```python
from build123d import *

# Parameters (mm, degrees)
SKETCH030_R             = 10
SKETCH030_R_2           = 1.55
SKETCH030_R_3           = 1.25
PAD027_DEPTH            = 2.5
SKETCH031_R             = 4.5
SKETCH031_R_2           = 3
PAD028_DEPTH            = 2
SKETCH032_R             = 3
POCKET009_DEPTH         = 1
BODY011_PLACEMENT_ANGLE = 180


with BuildPart() as part:
    # Sketch030 → Pad027 (new body)
    with BuildSketch(Plane.YZ):
        Circle(SKETCH030_R)
        Circle(SKETCH030_R_2, mode=Mode.SUBTRACT)
        with Locations((-7.35, 0)):
            Circle(SKETCH030_R_3, mode=Mode.SUBTRACT)
        with Locations((0, -7.35)):
            Circle(SKETCH030_R_3, mode=Mode.SUBTRACT)
        with Locations((7.35, 0)):
            Circle(SKETCH030_R_3, mode=Mode.SUBTRACT)
        with Locations((0, 7.35)):
            Circle(SKETCH030_R_3, mode=Mode.SUBTRACT)
    extrude(amount=PAD027_DEPTH)

    # Sketch031 (on Face8 of Pad027) → Pad028 (join)
    with BuildSketch(Plane.YZ.offset(2.5)):
        Circle(SKETCH031_R)
        Circle(SKETCH031_R_2, mode=Mode.SUBTRACT)
    extrude(amount=PAD028_DEPTH)

    # Sketch032 (on Face10 of Pad028) → Pocket009 (cut)
    with BuildSketch(Plane.YZ.offset(2.5)):
        Circle(SKETCH032_R)
    extrude(amount=-POCKET009_DEPTH, mode=Mode.SUBTRACT)


with BuildPart() as part_1:
    # Body011 placement: moved
    add(part.part.moved(Location((19.2, 11.3, 0))).rotate(Axis((19.2, 11.3, 0), (0, 0, 1)), BODY011_PLACEMENT_ANGLE))


solid = part_1.part
```
Design review of the part built by this model. Coordinates are the model's own, in mm. Coordinates: 2 decimals unless noted, no trailing zeros. Write each loop counter-clockwise with the first axis right and the second up, starting at its lowest first coordinate (ties: lowest second). Pieces come first, ordered by that corner, then holes.
1) Insertion check: pin 1 (4 mm diameter, centred on y = 11.3, z = 7.35, fed in from -X); pin 2 (1.8 mm diameter, centred on y = 11.5, z = 0.5, fed in from -X); pin 3 (1 mm diameter, centred on x = 18, z = -7, fed in from +Y). Each pin has a flat end and moves straight along its axis. Give the tip position at first contact, or say it passes through.
2) Add section D-D (z = 7.35). Write out the cut boundary in (x, y).
3) Add section B-B (y = 11.3). Write out the cut boundary in (x, z), plus the area to 4 significant figures.
4) Add section C-C (y = 3.95). Write out the cut boundary in (x, z).
5) Add section A-A (z = 0). Write out the cut boundary in (x, y).
6) To check wall thickness, follow L1, parallel to Z at x = 17.3, y = 11.3; L2, parallel to Y at x = 18.45, z = 1; L3, parallel to X at y = 8, z = 6. State the ranges of each line that lie inside material, in increasing order.
7) Mouldability with a two-part tool opening along Y and no side actions: class faces 1 (the cylindrical face through (15.714, 15.796, 0.198)), 2 (the flat face through (16.7, 7, -2)), 3 (the flat face through (17.7, 10, -1.3)) as +Y half, -Y half, draft (parallel to the pull), parting line (faces both ways), or undercut.
Check result:
1. pin 1: stops at x = 16.7
1. pin 2: passes through
1. pin 3: stops at y = 18.9
2. outline: (16.7, 4.52) - (19.2, 4.52) - (19.2, 10.05) - (16.7, 10.05) - close; (16.7, 12.55) - (19.2, 12.55) - (19.2, 18.08) - (16.7, 18.08) - close
3. outline: (14.7, -4.5) - (16.7, -4.5) - (16.7, -6.1) - (19.2, -6.1) - (19.2, -1.55) - (17.7, -1.55) - (17.7, -3) - (14.7, -3) - close; (14.7, 3) - (17.7, 3) - (17.7, 1.55) - (19.2, 1.55) - (19.2, 6.1) - (16.7, 6.1) - (16.7, 4.5) - (14.7, 4.5) - close; (16.7, -10) - (19.2, -10) - (19.2, -8.6) - (16.7, -8.6) - close; (16.7, 8.6) - (19.2, 8.6) - (19.2, 10) - (16.7, 10) - close
3. area: 32.85 mm2
4. outline: (16.7, -6.78) - (19.2, -6.78) - (19.2, -1.25) - (16.7, -1.25) - close; (16.7, 1.25) - (19.2, 1.25) - (19.2, 6.78) - (16.7, 6.78) - close
5. outline: (14.7, 6.8) - (16.7, 6.8) - (16.7, 5.2) - (19.2, 5.2) - (19.2, 9.75) - (17.7, 9.75) - (17.7, 8.3) - (14.7, 8.3) - close; (14.7, 14.3) - (17.7, 14.3) - (17.7, 12.85) - (19.2, 12.85) - (19.2, 17.4) - (16.7, 17.4) - (16.7, 15.8) - (14.7, 15.8) - close; (16.7, 1.3) - (19.2, 1.3) - (19.2, 2.7) - (16.7, 2.7) - close; (16.7, 19.9) - (19.2, 19.9) - (19.2, 21.3) - (16.7, 21.3) - close
6. L1: z = -10 to -8.6, -6.1 to -3, 3 to 6.1, 8.6 to 10
6. L2: y = 1.35 to 3.2, 4.7 to 10.12, 12.48 to 17.9, 19.4 to 21.25
6. L3: x = 16.7 to 19.2
7. face 1: parting line
7. face 2: draft
7. face 3: undercut
